Here's how the part is built. I have some questions about the finished solid (model axes, mm). Give positions to 0.01 mm unless a question says otherwise; leave off trailing zeros. Loops run counter-clockwise (first coordinate to the right, second up) from the corner with the lowest first, then second, coordinate; pieces in that order, holes last.
Q1. Suppose I cut it at A-A (x = 90). List the corners of the cut face in (y, z) for me.
Q2. I need wall thicknesses on probe 1 along Y at (x, z) = (15, 0.75); probe 2 along Y at (x, z) = (12.5, 0.7); probe 3 along Y at (x, z) = (7, 0.85). Which ranges of each line are inside material? Lowest first, please.
Q3. Suppose I cut it at B-B (z = 0.55). Count the separate pieces of the cut face and the enclosed holes in it, and give its area (3 significant figures).
Q4. Suppose I cut it at C-C (y = 28). List the corners of the cut face in (x, z) for me, and give its area (3 significant figures).
Q5. Suppose I cut it at D-D (y = 5). List the corners of the cut face in (x, z) for me.
Q6. I'm going to push a flat-ended pin straight in: P1, Ø1.2, axis at x = 15, y = 19.5, coming from the -Z side. Where does the tip first touch, or does it pass through?
```python
from build123d import *

# Parameters (mm, degrees)
ESQUISSE1_W                                 = 100
ESQUISSE1_H                                 = 100
BOSS_EXTRU_1_DEPTH                          = 1
FRAISAGE_POUR_VIS_T_TE_FRAIS_E_M31_AT_COUNT = 2
FRAISAGE_POUR_VIS_T_TE_FRAIS_E_M31_AT_PITCH = 90
FRAISAGE_POUR_VIS_T_TE_FRAIS_E_M31_2_COUNT  = 2
FRAISAGE_POUR_VIS_T_TE_FRAIS_E_M31_2_PITCH  = 127.279220614
FRAISAGE_POUR_VIS_T_TE_FRAIS_E_M31_3_COUNT  = 2
FRAISAGE_POUR_VIS_T_TE_FRAIS_E_M31_3_PITCH  = 90
ESQUISSE4_R                                 = 5.05
ESQUISSE4_R_2                               = 1
ENL_V_MAT_EXTRU_1_DEPTH                     = 2


with BuildPart() as part:
    # Esquisse1 → Boss.-Extru.1 (new body)
    with BuildSketch(Plane.XY):
        with Locations((50, 50)):
            Rectangle(ESQUISSE1_W, ESQUISSE1_H)
    extrude(amount=BOSS_EXTRU_1_DEPTH)

    # Esquisse3 → Fraisage pour vis à tête fraisée M31 (revolve, cut)
    with BuildSketch(Plane(origin=(5, 95, 1), x_dir=(0, -1, 0), z_dir=(1, 0, 0))):
        Polygon((0, 0), (0, 1), (1.8, 1), (1.8, 1.35), (3.15, 0), align=None)
    fraisage_pour_vis_t_te_frais_e_m31 = revolve(axis=Axis((5, 95, 7.35), (0, 0, -1)), mode=Mode.SUBTRACT)

    # Fraisage pour vis à tête fraisée M31 at: Fraisage pour vis à tête fraisée M31 ×2
    with Locations(*[(i * FRAISAGE_POUR_VIS_T_TE_FRAIS_E_M31_AT_PITCH, 0, 0) for i in range(1, FRAISAGE_POUR_VIS_T_TE_FRAIS_E_M31_AT_COUNT)]):
        add(fraisage_pour_vis_t_te_frais_e_m31, mode=Mode.SUBTRACT)

    # Fraisage pour vis _ t_te frais_e M31 2: Fraisage pour vis à tête fraisée M31 ×2
    with Locations(*[Vector(0.707106781, -0.707106781, 0) * (i * FRAISAGE_POUR_VIS_T_TE_FRAIS_E_M31_2_PITCH) for i in range(1, FRAISAGE_POUR_VIS_T_TE_FRAIS_E_M31_2_COUNT)]):
        add(fraisage_pour_vis_t_te_frais_e_m31, mode=Mode.SUBTRACT)

    # Fraisage pour vis _ t_te frais_e M31 3: Fraisage pour vis à tête fraisée M31 ×2
    with Locations(*[(0, -i * FRAISAGE_POUR_VIS_T_TE_FRAIS_E_M31_3_PITCH, 0) for i in range(1, FRAISAGE_POUR_VIS_T_TE_FRAIS_E_M31_3_COUNT)]):
        add(fraisage_pour_vis_t_te_frais_e_m31, mode=Mode.SUBTRACT)

    # Esquisse4 → Enlèv. mat.-Extru.1 (cut, through all)
    with BuildSketch(Plane.XY.offset(1)):
        with Locations((90, 28)):
            Circle(ESQUISSE4_R)
        with Locations((12.5, 25)):
            Circle(ESQUISSE4_R_2)
        with Locations((10, 19.5)):
            Circle(ESQUISSE4_R_2)
        with Locations((7, 25)):
            Circle(ESQUISSE4_R_2)
        with Locations((18, 25)):
            Circle(ESQUISSE4_R_2)
        with Locations((10, 30.5)):
            Circle(ESQUISSE4_R_2)
        with Locations((15, 30.5)):
            Circle(ESQUISSE4_R_2)
        with Locations((15, 19.5)):
            Circle(ESQUISSE4_R_2)
    extrude(amount=-ENL_V_MAT_EXTRU_1_DEPTH, mode=Mode.SUBTRACT)


solid = part.part
```
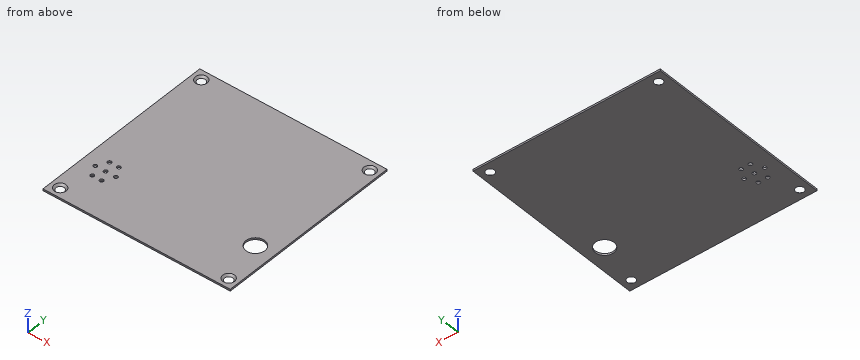
Solutions:
1. outline: (0, 0) - (22.95, 0) - (22.95, 1) - (0, 1) - close; (33.05, 0) - (100, 0) - (100, 1) - (33.05, 1) - close
2. probe 1: y = 0 to 18.5, 20.5 to 29.5, 31.5 to 100
2. probe 2: y = 0 to 24, 26 to 100
2. probe 3: y = 0 to 2.76, 7.24 to 24, 26 to 92.76, 97.24 to 100
3. separate pieces: 1
3. enclosed holes: 12
3. area: 9,810 mm2
4. outline: (0, 0) - (84.95, 0) - (84.95, 1) - (0, 1) - close; (95.05, 0) - (100, 0) - (100, 1) - (95.05, 1) - close
4. area: 89.9 mm2
5. outline: (0, 0) - (2.85, 0) - (1.85, 1) - (0, 1) - close; (7.15, 0) - (92.85, 0) - (91.85, 1) - (8.15, 1) - close; (97.15, 0) - (100, 0) - (100, 1) - (98.15, 1) - close
6. P1: passes through
